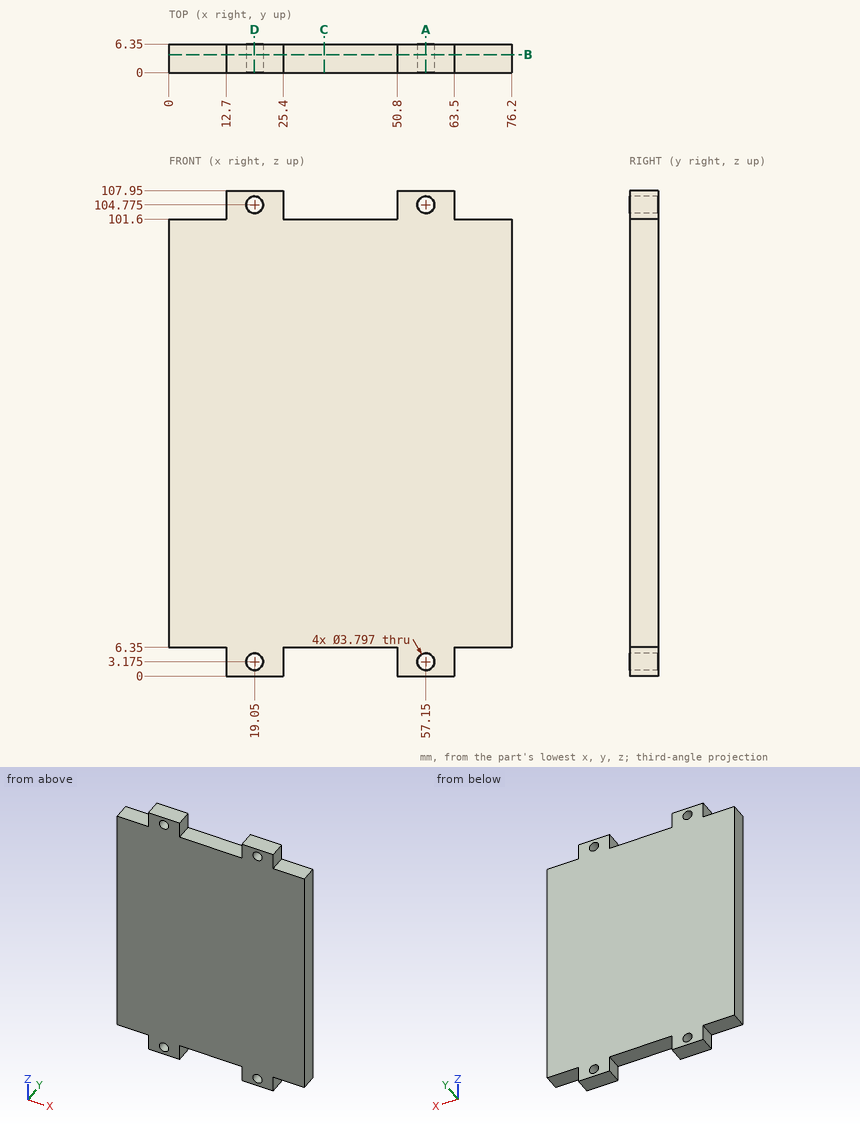
Source: three-view drawing plus pictorial views. Frame: mm from the lowest corner of the part. Coordinates: 2 decimals unless noted, no trailing zeros. Order: outer loops, then holes, each group sorted by start corner. A loop starts at its lowest first (then second) coordinate and runs counter-clockwise, first axis right, second up.
1) Section B-B (y = 4). Give the number of separate pieces and of enclosed holes in the cut face, then the cut area to 3 significant figures.
Result sheet:
separate pieces: 1
enclosed holes: 4
area: 7,540 mm2
2) Section A-A (x = 57.15). Return loops of the section in (y, z), then the cut area to 3 significant figures.
Result sheet:
outline: (0, 0) - (6.35, 0) - (6.35, 1.28) - (0, 1.28) - close; (0, 5.07) - (6.35, 5.07) - (6.35, 102.88) - (0, 102.88) - close; (0, 106.67) - (6.35, 106.67) - (6.35, 107.95) - (0, 107.95) - close
area: 637 mm2
3) First-contact query: P1, Ø3, axis at x = 38, y = 4.5, coming from the -Z side; P2, Ø3, axis at x = 69, y = 4, coming from the +Z side. Flat tips, straight axial feed; report the tip coordinate or a pass-through.
Result sheet:
P1: stops at z = 6.35
P2: stops at z = 101.6
4) Ray query, probe 1 along Z at (x, y) = (19.05, 2.75); probe 2 along Z at (x, y) = (26.5, 4.5). Return the intervals inside material, ascending.
Result sheet:
probe 1: z = 0 to 1.28, 5.07 to 102.88, 106.67 to 107.95
probe 2: z = 6.35 to 101.6
5) Section C-C (x = 34.5). Return loops of the section in (y, z), then the cut area to 3 significant figures.
Result sheet:
outline: (0, 6.35) - (6.35, 6.35) - (6.35, 101.6) - (0, 101.6) - close
area: 605 mm2
